```python
from build123d import *

# Parameters (mm, degrees)
SKETCH2_R           = 11
BOSS_EXTRUDE1_DEPTH = 7.5
SKETCH5_R           = 1.984375
CUT_EXTRUDE3_DEPTH  = 74.683320442
CIRPATTERN1_COUNT   = 3
SKETCH6_R           = 1.675
CUT_EXTRUDE4_DEPTH  = 70.030252146


with BuildPart() as part:
    # Sketch2 → Boss-Extrude1 (new body)
    with BuildSketch(Plane.XY):
        Polygon((-25, 0), (25, 0), (25, 5), (19, 5), (19, 68.9056), (-19, 68.9056), (-19, 5), (-25, 5), align=None)
        with Locations((0, 48.9056)):
            Circle(SKETCH2_R, mode=Mode.SUBTRACT)
    extrude(amount=-BOSS_EXTRUDE1_DEPTH)

    # Sketch5 → Cut-Extrude3 (cut, through all)
    with BuildSketch(Plane.XY):
        with Locations((0, 63.9056)):
            Circle(SKETCH5_R)
    cut_extrude3 = extrude(amount=-CUT_EXTRUDE3_DEPTH, mode=Mode.SUBTRACT)

    # CirPattern1: Cut-Extrude3 ×3 about axis
    cirpattern1_axis = Axis((0, 48.9056, 0), (0, 0, 1))
    for i in range(1, CIRPATTERN1_COUNT):
        add(cut_extrude3.rotate(cirpattern1_axis, i * 360 / CIRPATTERN1_COUNT), mode=Mode.SUBTRACT)

    # Sketch6 → Cut-Extrude4 (cut, through all)
    with BuildSketch(Plane(origin=(0, 5, 0), x_dir=(1, 0, 0), z_dir=(0, 1, 0))):
        with Locations(Location((22, 3.75, 0), (0, 0, 270))):
            Circle(SKETCH6_R)
        with Locations(Location((-22, 3.75, 0), (0, 0, 270))):
            Circle(SKETCH6_R)
    extrude(amount=-CUT_EXTRUDE4_DEPTH, mode=Mode.SUBTRACT)


solid = part.part
```
Work out the finished part from the listing and answer in its coordinate system (mm). A direction names the side the tool comes from. Round coordinates to 2 decimals unless told otherwise and drop trailing zeros. Write each loop counter-clockwise with the first axis right and the second up, starting at its lowest first coordinate (ties: lowest second). Pieces come first, ordered by that corner, then holes.
1) A cutting plane is placed at B-B on z = -3.75. Determine the outline of the cut face in (x, y) (3 decimals), and give its area (3 significant figures).
2) Determine the mould class of faces 1 (the face through (25, 2, -4)), 2 (the face through (0, 27, -7.5)), 3 (the face through (-25, 3, -4)), 4 (the face through (12.732, 43.373, -3.698)) for opening direction X: pulls with the +X half, pulls with the -X half, needs draft (parallel to the pull), parting line crosses it, or undercut.
3) A cutting plane is placed at A-A on x = 0. Determine the outline of the cut face in (y, z), and give its area (3 significant figures).
4) Consider probe 1 along X at (y, z) = (1.45, -3.75) (3 decimals); probe 2 along Y at (x, z) = (0, -0.5); probe 3 along Y at (x, z) = (0.5, -3). Determine where each line is inside the solid, lowest interval first.
5) A cutting plane is placed at C-C on x = -22. Determine the outline of the cut face in (y, z) (3 decimals), and give its area (4 significant figures).
6) Flat-ended cylindrical pins translate along their axes: P1, Ø3, axis at x = 22, z = -3.75, coming from the +Y side; P2, Ø1.8, axis at x = 22.5, z = -2, coming from the +Y side; P3, Ø3, axis at y = 20, z = -3.5, coming from the +X side. Find the tip coordinate at first contact, or state that the pin passes through.
7) A cutting plane is placed at D-D on y = 32. Determine the outline of the cut face in (x, z).
8) Which of the six approach directions +Z, -Z, +X, -X, +Y, -Y give full straight-line access (tool end or side, diameter ignored) to faces 5 (the face through (-21, 5, -2)), 6 (the face through (21, 5, -2)), 7 (the face through (0, 0, -4))?
Entries:
1. outline: (-25, 0) - (-23.675, 0) - (-23.675, 5) - (-25, 5) - close; (-20.325, 0) - (20.325, 0) - (20.325, 5) - (19, 5) - (19, 68.906) - (-19, 68.906) - (-19, 5) - (-20.325, 5) - close; (23.675, 0) - (25, 0) - (25, 5) - (23.675, 5) - close; hole circle Ø3.969 at (-12.99, 41.406); hole circle Ø22 at (0, 48.906); hole circle Ø3.969 at (0, 63.906); hole circle Ø3.969 at (12.99, 41.406)
1. area: 2,230 mm2
2. face 1: pulls with the +X half
2. face 2: needs draft
2. face 3: pulls with the -X half
2. face 4: undercut
3. outline: (0, -7.5) - (37.91, -7.5) - (37.91, 0) - (0, 0) - close; (59.91, -7.5) - (61.92, -7.5) - (61.92, 0) - (59.91, 0) - close; (65.89, -7.5) - (68.91, -7.5) - (68.91, 0) - (65.89, 0) - close
3. area: 322 mm2
4. probe 1: x = -25 to -23.675, -20.325 to 20.325, 23.675 to 25
4. probe 2: y = 0 to 37.91, 59.91 to 61.92, 65.89 to 68.91
4. probe 3: y = 0 to 37.92, 59.89 to 61.99, 65.83 to 68.91
5. outline: (0, -7.5) - (5, -7.5) - (5, -5.425) - (0, -5.425) - close; (0, -2.075) - (5, -2.075) - (5, 0) - (0, 0) - close
5. area: 20.75 mm2
6. P1: passes through
6. P2: stops at y = 5
6. P3: stops at x = 19
7. outline: (-19, -7.5) - (19, -7.5) - (19, 0) - (-19, 0) - close
8. face 5: +Z, -Z, -X, +Y
8. face 6: +Z, -Z, +X, +Y
8. face 7: +Z, -Z, +X, -X, -Y
